```python
from build123d import *

# Parameters (mm, degrees)
SKETCH1_W           = 14.5
SKETCH1_H           = 49.5
BOSS_EXTRUDE1_DEPTH = 70
FILLET1_R           = 10
SKETCH2_R           = 5
CUT_EXTRUDE1_DEPTH  = 76.649272964
BOSS_EXTRUDE2_DEPTH = 8
SKETCH5_R           = 1.7
CUT_EXTRUDE2_DEPTH  = 15
CUT_EXTRUDE3_DEPTH  = 5
CUT_EXTRUDE4_DEPTH  = 103.041964407
CUT_EXTRUDE5_DEPTH  = 10
FILLET2_R           = 1.5
FILLET3_R           = 3
SKETCH10_R          = 2.2
CUT_EXTRUDE6_DEPTH  = 19.5
SKETCH11_R          = 1.7
CUT_EXTRUDE7_DEPTH  = 3


with BuildPart() as part:
    # Sketch1 → Boss-Extrude1 (new body)
    with BuildSketch(Plane(origin=(0, 0, 0), x_dir=(1, 0, 0), z_dir=(0, 1, 0))):
        Rectangle(SKETCH1_W, SKETCH1_H)
    extrude(amount=BOSS_EXTRUDE1_DEPTH)

    # Fillet1
    fillet1_edges = [part.edges().sort_by_distance(p)[0] for p in [
        (0, 0, 24.75),
        (0, 0, -24.75),
    ]]
    fillet(fillet1_edges, radius=FILLET1_R)

    # Sketch2 → Cut-Extrude1 (cut, through all)
    with BuildSketch(Plane(origin=(7.25, 0, 0), x_dir=(0, 0, -1), z_dir=(1, 0, 0))):
        with Locations((-12, 7)):
            Circle(SKETCH2_R)
        with Locations(Location((12, 7, 0), (0, 0, 180))):
            Circle(SKETCH2_R)
    extrude(amount=-CUT_EXTRUDE1_DEPTH, mode=Mode.SUBTRACT)

    # Sketch3 → Boss-Extrude2 (add)
    with BuildSketch(Plane(origin=(0, 70, 0), x_dir=(1, 0, 0), z_dir=(0, 1, 0))):
        Polygon((77.25, 8.5), (77.25, -8.5), (7.25, -24.75), (7.25, 24.75), align=None)
    extrude(amount=-BOSS_EXTRUDE2_DEPTH)

    # Sketch5 → Cut-Extrude2 (cut)
    with BuildSketch(Plane(origin=(77.25, 0, 0), x_dir=(0, 0, -1), z_dir=(1, 0, 0))):
        with Locations((-4.25, 66)):
            Circle(SKETCH5_R)
        with Locations((4.25, 66)):
            Circle(SKETCH5_R)
    extrude(amount=-CUT_EXTRUDE2_DEPTH, mode=Mode.SUBTRACT)

    # Sketch7 → Cut-Extrude3 (cut)
    with BuildSketch(Plane(origin=(62.25, 0, 0), x_dir=(0, 0, -1), z_dir=(1, 0, 0))):
        Polygon((-7.5, 66), (-7.5, 70), (-1, 70), (-1, 66), (-2.625, 63.185417438), (-5.875, 63.185417438), align=None)
        Polygon((1, 66), (2.625, 63.185417438), (5.875, 63.185417438), (7.5, 66), (7.5, 70), (1, 70), align=None)
    extrude(amount=CUT_EXTRUDE3_DEPTH, mode=Mode.SUBTRACT)

    # Sketch8 → Cut-Extrude4 (cut, through all)
    with BuildSketch(Plane(origin=(7.25, 0, 0), x_dir=(0, 0, -1), z_dir=(1, 0, 0))):
        Polygon((0.021408878, 36.140810628), (15.98032373, 22), (-15.533482813, 22), align=None)
        Polygon((-19.75, 24.924106533), (-19.75, 53.65978052), (-3.742755965, 39.476146565), align=None)
        Polygon((-15.98032373, 57), (15.533482813, 57), (-0.021408878, 42.859189372), align=None)
        Polygon((19.75, 25.34021948), (19.75, 54.075893467), (3.742755965, 39.523853435), align=None)
    extrude(amount=-CUT_EXTRUDE4_DEPTH, mode=Mode.SUBTRACT)

    # Sketch9 → Cut-Extrude5 (cut)
    with BuildSketch(Plane(origin=(0, 70, 0), x_dir=(1, 0, 0), z_dir=(0, 1, 0))):
        Polygon((35.452952842, 0), (12.25, -16.025665333), (12.25, 16.025665333), align=None)
        Polygon((49.616038971, 9.782068685), (17.550981037, 17.225742848), (38.972216713, 2.430662399), align=None)
        Polygon((57.25, 10.193318694), (42.491480584, 0), (57.25, -10.193318694), align=None)
        Polygon((38.972216713, -2.430662399), (49.616038971, -9.782068685), (17.550981037, -17.225742848), align=None)
    extrude(amount=-CUT_EXTRUDE5_DEPTH, mode=Mode.SUBTRACT)

    # Fillet2
    fillet2_edges = [part.edges().sort_by_distance(p)[0] for p in [
        (57.25, 66, -10.193318694),
        (57.25, 66, 10.193318694),
    ]]
    fillet(fillet2_edges, radius=FILLET2_R)

    # Fillet3
    fillet3_edges = [part.edges().sort_by_distance(p)[0] for p in [
        (7.25, 62, 0),
    ]]
    fillet(fillet3_edges, radius=FILLET3_R)

    # Sketch10 → Cut-Extrude6 (cut)
    with BuildSketch(Plane.ZY.offset(7.25)):
        with Locations((-9.75, 65.5)):
            Circle(SKETCH10_R)
        with Locations((9.898872111, 65.837689232)):
            Circle(SKETCH10_R)
    extrude(amount=-CUT_EXTRUDE6_DEPTH, mode=Mode.SUBTRACT)

    # Sketch11 → Cut-Extrude7 (cut)
    with BuildSketch(Plane(origin=(62.25, 0, 0), x_dir=(0, 0, -1), z_dir=(1, 0, 0))):
        with Locations((4.25, 66)):
            Circle(SKETCH11_R)
        with Locations((-4.25, 66)):
            Circle(SKETCH11_R)
    extrude(amount=-CUT_EXTRUDE7_DEPTH, mode=Mode.SUBTRACT)


solid = part.part
```
Read the model definition and answer for the solid it produces. Units are mm, in the model's axes. A direction names the side the tool comes from. Give positions to 0.01 mm unless a question says otherwise; leave off trailing zeros. Loops run counter-clockwise (first coordinate to the right, second up) from the corner with the lowest first, then second, coordinate; pieces in that order, holes last.
Item 1: The part is cut by section A-A (y = 31). Write down the section's boundary in (x, z).
Item 2: Find the intervals of material crossed by line 1 along Y through (x, z) = (70, -4.25); line 2 along Y through (x, z) = (-3, -6); line 3 along Z through (x, y) = (61, 66), in increasing order.
Item 3: The mould has two halves that part along X. Classify faces 1 (the flat face through (-7.25, 35, -5)), 2 (the flat face through (59.25, 66, -4)), 3 (the flat face through (65, 68, -1)), 4 (the cylindrical face through (2.36, 63.69, 9.42)): released by +X, released by -X, zero draft, split by the parting line, or undercut.
Item 4: The part is cut by section D-D (y = 7). Write down the section's boundary in (x, z).
Item 5: The part is cut by section B-B (x = 65). Write down the section's boundary in (y, z) (3 decimals), and give its area (3 significant figures).
Item 6: Each of these flat-tipped pins is pushed along its axis until it touches: pin 1 Ø6 at (x, y) = (66, 61.5) entering from +Z; pin 2 Ø2 at (x, y) = (65.5, 67.5) entering from +Z; pin 3 Ø4 at (y, z) = (65.5, -9.75) entering from -X; pin 4 Ø12 at (x, y) = (19, 20.5) entering from +Z. Where does it stop, or does it pass through?
Item 7: The part is cut by section C-C (z = 13.5). Give the number of separate pieces and of enclosed holes in the cut face, and give its area (3 significant figures).
Item 8: For faces 5 (the cylindrical face through (2.364, 67.355, -8.567)), 6 (the flat face through (65, 68, 7.5)), 7 (the flat face through (7.25, 16, 0)), determine the directions among +Z, -Z, +X, -X, +Y, -Y from which every point of the face is accessible in a straight line to the end or side of a thin tool.
Taken from the geometry:
1. outline: (-7.25, -24.75) - (7.25, -24.75) - (7.25, -19.75) - (-7.25, -19.75) - close; (-7.25, -13.36) - (7.25, -13.36) - (7.25, -5.82) - (-7.25, -5.82) - close; (-7.25, 5.63) - (7.25, 5.63) - (7.25, 13.07) - (-7.25, 13.07) - close; (-7.25, 19.75) - (7.25, 19.75) - (7.25, 24.75) - (-7.25, 24.75) - close
2. line 1: y = 62 to 64.3, 67.7 to 70
2. line 2: y = 0 to 22, 30.84 to 37.52, 41.58 to 48.33, 57 to 70
2. line 3: z = -12.27 to -5.95, -2.55 to 2.55, 5.95 to 12.27
3. face 1: released by -X
3. face 2: released by +X
3. face 3: undercut
3. face 4: zero draft
4. outline: (-7.25, -24.29) - (7.25, -24.29) - (7.25, -17) - (-7.25, -17) - close; (-7.25, -7) - (7.25, -7) - (7.25, 7) - (-7.25, 7) - close; (-7.25, 17) - (7.25, 17) - (7.25, 24.29) - (-7.25, 24.29) - close
5. outline: (62, -11.344) - (70, -11.344) - (70, -7.5) - (66, -7.5) - (63.185, -5.875) - (63.185, -2.625) - (66, -1) - (70, -1) - (70, 1) - (66, 1) - (63.185, 2.625) - (63.185, 5.875) - (66, 7.5) - (70, 7.5) - (70, 11.344) - (62, 11.344) - close
5. area: 102 mm2
6. pin 1: stops at z = 11.8
6. pin 2: stops at z = 11.46
6. pin 3: stops at x = 18.44
6. pin 4: passes through
7. separate pieces: 7
7. enclosed holes: 0
7. area: 839 mm2
8. face 5: -X
8. face 6: +Y
8. face 7: +Z, -Z, +X, -Y
